Autodesk Inventor part; units mm, degrees
ref_plane "YZ Plane" through (0, 0, 0) normal (1, 0, 0) x (0, 1, 0)
ref_plane "XZ Plane" through (0, 0, 0) normal (0, 1, 0) x (-1, 0, 0)
ref_plane "XY Plane" through (0, 0, 0) normal (0, 0, 1) x (1, 0, 0)
sketch "Skizze1" plane through (0, 0, 0) normal (0, 1, 0) x (-1, 0, 0)
  arc A0 (12.3985, 1.5897) -> (0, 12.5) centre (0, 0) ccw
  line L0 (0, -34.7678) -> (0, 23.1071) construction
  line L1 (12.3985, 1.5897) -> (16, -26.5)
  line L2 (16, -26.5) -> (0, -26.5)
  arc A1 (0, 12.5) -> (-12.3985, 1.5897) centre (0, 0) ccw
  line L3 (-12.3985, 1.5897) -> (-16, -26.5)
  line L4 (-16, -26.5) -> (0, -26.5)
  line L5 (15.4871, -22.5) -> (-15.4871, -22.5)
  dimension "d0" = 25
  dimension "d1" = 32
  dimension "d2" = 39
  dimension "d3" = 35
extrude "Extrusion1" add sketch "Skizze1" along normal blind 9.5 contours L1 L5 L3 A1 A0
hole "Bohrung1" at (0, 0, 0) direction (0, 1, 0) diameter 4 depth 9.5
sketch "Skizze2" plane through (0, 9.5, 0) normal (0, 1, 0) x (1, 0, 0)
  line L0 (0, 29.5) -> (0, -19.5)
  arc A0 (-5, 0) -> (0, -5) centre (0, 0) ccw
  line L1 (-21.682, 0) -> (21.682, 0)
  circle A1 centre (0, 0) radius 2
  line L2 (0, -5) -> (0, -2)
  line L3 (-2, 0) -> (-5, 0)
  point P0 (0, 5)
  dimension "d6" = 10
revolve "Umdrehung1" add sketch "Skizze2" angle 180 about axis through (0, 9.5, 0) along (0, 0, -1) contours L0 A0 L1 A1
fillet "Rundung1" radius 1.5 4 edges at (-1.4142, 9.5, -1.4142) (1.4142, 9.5, -1.4142) (-1.4142, 9.5, 1.4142) (1.4142, 9.5, 1.4142)
sketch "Skizze3" plane through (15.4871, 0, -22.5) normal (0, 0, -1) x (-1, 0, 0)
  line L0 (0, 0) -> (30.9743, 0)
  line L1 (30.9743, 0) -> (30.9743, 9.5)
  line L2 (0, 9.5) -> (30.9743, 9.5)
  line L3 (0, 0) -> (0, 9.5)
  line L4 (3.0886, 9.5) -> (0, 9.5)
  line L5 (0, 9.5) -> (30.9743, 0) construction
  line L6 (30.9743, 9.5) -> (0, 0) construction
  point P0 (15.4871, 0)
  point P1 (15.4871, 4.75)
hole "Bohrung2" at (0, 4.75, -22.5) direction (0, 0, 1) diameter 3 end up to surface counterbore diameter 6 counterbore depth 7
properties part number "Steitenteil_kabel"
Source: CAD feature listing. Evaluate the final solid. Frame: model axes, mm. A direction names the side the tool comes from. Round coordinates to 2 decimals unless told otherwise and drop trailing zeros. Loops run counter-clockwise (first coordinate to the right, second up) from the corner with the lowest first, then second, coordinate; pieces in that order, holes last. Notation, with made-up numbers: M 72,-30 L 121,-30 A15 cw 121,-3 Z; hole C -6.75,23.5 d1. An arc over 180 degrees is marked long. Return JSON: item names as keys, results as strings. Group by question number.
1. Reachability of faces 4 (the face through (0, 5, 2)), 5 (the face through (0.575, 6.136, -8.312)), 6 (the face through (13.92, 4.68, -10.29)) from +Z, -Z, +X, -X, +Y, -Y: full face, straight path, thin tool, end or side. Return the list, or none.
2. Material intervals for line 1 along Y through (x, z) = (0, -7); line 2 along Y through (x, z) = (11, -18); line 3 along X through (y, z) = (3.5, 0), sorted ascending. Write a range as from..to.
3. Section query B-B on z = -5. Output: boundary loops of the cut face in (x, y).
4. Section query C-C on x = 10. Output: boundary loops of the cut face in (y, z), and give its area (3 significant figures).
5. Section query A-A on y = 4.75. Output: boundary loops of the cut face in (x, z), and give its area (3 significant figures).
6. Mould query, pull axis Y, two halves, no side actions, for faces 1 (the face through (0, 12, 0)), 2 (the face through (1, 3, -15.5)), 3 (the face through (0, 0, -9)). Classes: released by +Y, released by -Y, zero draft, split by the parting line, or undercut.
7. Section query D-D on z = 4. Output: boundary loops of the cut face in (x, y).
8. Pin query (flat end, axial travel): pin 1 (2 mm diameter, centred on x = -4, z = -10, fed in from +Y); pin 2 (4 mm diameter, centred on y = 3.5, z = 0, fed in from +X); pin 3 (1.8 mm diameter, centred on x = 0.5, y = 5.5, fed in from -Z). Return the tip coordinate at first contact, or that it passes through.
Checks:
{
 "1": {"face 4": "-Y", "face 5": "-Z", "face 6": "+Z, +X, +Y, -Y"},
 "2": {"line 1": "y = 0..3.25, 6.25..9.5", "line 2": "y = 0..9.5", "line 3": "x = -12.6..-2, 2..12.6"},
 "3": {"outline": "M -13.24,0 L 13.24,0 L 13.24,9.5 L -13.24,9.5 Z; hole C 0,4.75 d3"},
 "4": {"outline": "M 0,-22.5 L 9.5,-22.5 L 9.5,7.5 L 0,7.5 Z", "area": "285 mm²"},
 "5": {"outline": "M -15.49,-22.5 L -3,-22.5 L -3,-15.5 L -1.5,-15.5 L -1.5,-1.32 A2 cw long 1.5,-1.32 L 1.5,-15.5 L 3,-15.5 L 3,-22.5 L 15.49,-22.5 L 12.4,1.59 A12.5 ccw 0,12.5 A12.5 ccw -12.4,1.59 Z", "area": "782 mm²"},
 "6": {"face 1": "zero draft", "face 2": "undercut", "face 3": "released by -Y"},
 "7": {"outline": "M -11.84,0 L 11.84,0 L 11.84,9.5 L 3,9.5 A3 ccw -3,9.5 L -11.84,9.5 Z"},
 "8": {"pin 1": "stops at y = 9.5", "pin 2": "stops at x = 12.86", "pin 3": "stops at z = -15.5"}
}
